For this review, use the dimensioned drawing (mm, ordinates from the lowest corner) and the shaded views. Coordinates: 2 decimals unless noted, no trailing zeros. Write each loop counter-clockwise with the first axis right and the second up, starting at its lowest first coordinate (ties: lowest second). Pieces come first, ordered by that corner, then holes. Notation, with made-up numbers: M -20.75,2 L -2.75,2 A34 ccw -2.75,33 Z; hole C 38,-36 d10. An arc over 180 degrees is marked long. One line per question, with ' | ' between items.
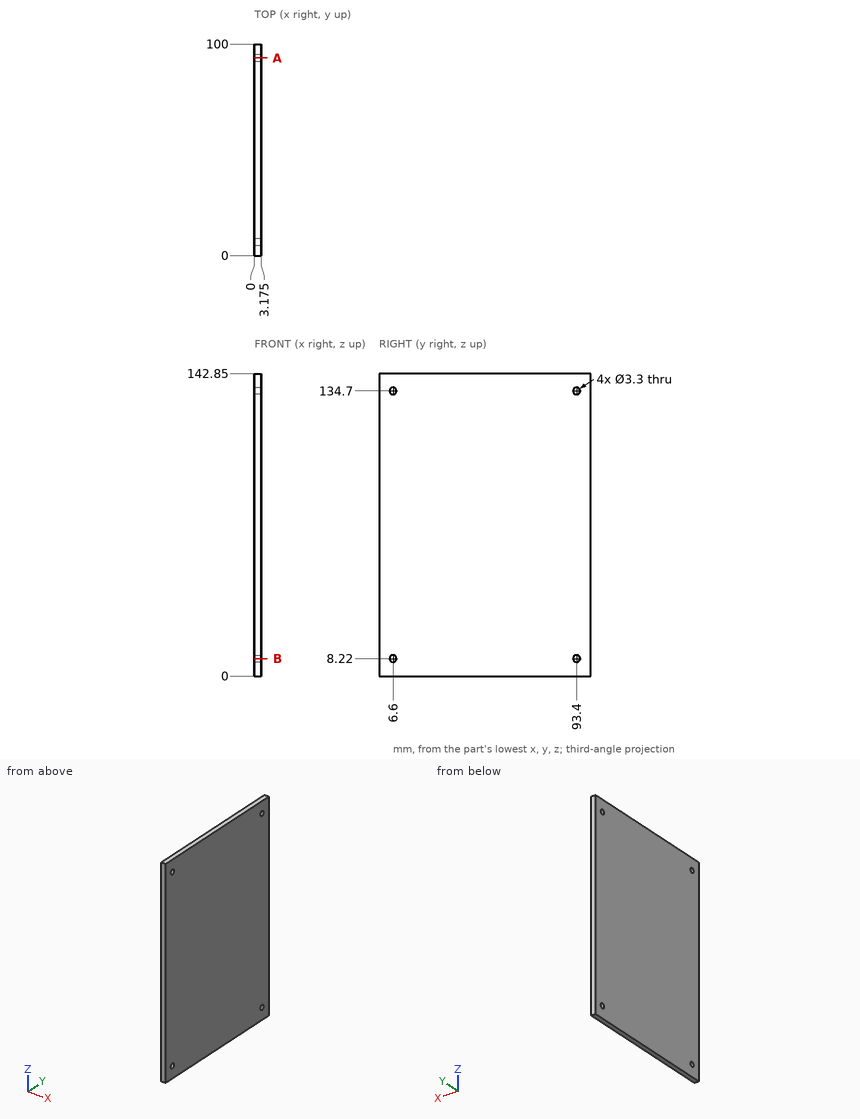
1. Take a section at A-A (y = 93.4). Write out the cut boundary in (x, z) (3 decimals), then the cut area to 3 significant figures.
Answer sheet:
outline: M 0,0 L 3.175,0 L 3.175,6.57 L 0,6.57 Z; M 0,9.87 L 3.175,9.87 L 3.175,133.05 L 0,133.05 Z; M 0,136.35 L 3.175,136.35 L 3.175,142.85 L 0,142.85 Z | area: 433 mm^2
2. Take a section at B-B (z = 8.22). Write out the cut boundary in (x, y) (3 decimals).
Answer sheet:
outline: M 0,0 L 3.175,0 L 3.175,4.95 L 0,4.95 Z; M 0,8.25 L 3.175,8.25 L 3.175,91.75 L 0,91.75 Z; M 0,95.05 L 3.175,95.05 L 3.175,100 L 0,100 Z
3. To check wall thickness, follow line 1 along Z through (x, y) = (1.5, 93.4); line 2 along Y through (x, z) = (1.1, 8.22); line 3 along Z through (x, y) = (0.3, 94). State the ranges of each line that lie inside material, in increasing order. Write a range as [from, to].
Answer sheet:
line 1: [0, 6.57], [9.87, 133.05], [136.35, 142.85] | line 2: [0, 4.95], [8.25, 91.75], [95.05, 100] | line 3: [0, 6.68], [9.76, 133.16], [136.24, 142.85]
